Design review of the part built by this model. Coordinates are the model's own, in mm. A direction names the side the tool comes from. Give positions to 0.01 mm unless a question says otherwise; leave off trailing zeros. Loops run counter-clockwise (first coordinate to the right, second up) from the corner with the lowest first, then second, coordinate; pieces in that order, holes last. Notation, with made-up numbers: M 11,24 L 26,24 A28 cw 26,49 Z; hole C 37.25,6 d5. An arc over 180 degrees is marked long. Use a Markdown table: item, result. Add a question column.
(1) Add section C-C, the plane x = 7. Give the boundary of the cut face in (y, z).
(2) For faces 1 (the face through (0.507, -2.1, 0.5)), 2 (the face through (0.1, 3.954, 0.5)), list the 3-axis set-ups (+Z, -Z, +X, -X, +Y, -Y) from which the entire face can be reached by the end or side of a thin tool; tool diameter is ignored.
(3) Add section A-A, the plane x = 4.75. Give the boundary of the cut face in (y, z).
(4) Add section B-B, the plane y = -2.25. State how many separate pieces and enclosed holes the cut face has, then the cut area to 3 significant figures.
(5) For probe 1 along Y at (x, z) = (1.5, 0.6); probe 2 along Y at (x, z) = (3.5, 0.15); probe 3 along X at (y, z) = (-2.25, 0.5), list the stretches that pass through material, from the lowest coordinate up.
(6) Add section D-D, the plane z = 0.6. Give the boundary of the cut face in (x, y), then the cut area to 3 significant figures.
(7) Insertion check: pin 1 Ø0.5 at (y, z) = (-2.5, 0.5) entering from +X. The pin has a flat end and moves straight along its axis. Give the tip position at first contact, or say it passes through.
(8) Draft analysis for pull direction X (two halves, no side actions). For faces 3 (the face through (4.425, 1.184, 0.493)), 4 (the face through (-1, 0, 1)), 5 (the face through (8.036, -0.039, 0.699)), state which applies: pulls with the +X half, pulls with the -X half, needs draft (parallel to the pull), parting line crosses it, or undercut.
```python
from build123d import *

# Parameters (mm, degrees)
F1_DEPTH = 1
F2_R     = 0.99999


# Not quite as in the source:
# - a fillet or chamfer is up to 0.001 mm smaller than in the source, because OpenCascade refuses the exact size


with BuildPart() as f1:
    # F0 (on Top) → F1 (new body)
    with BuildSketch(Plane.XY):
        Polygon((-7.3084038651, 2.5000789639), (-8.3084038651, 2.9543336025), (-8.3084038651, -3.1456663975), (-7.3084038651, -2.6904001687), align=None)
        Polygon((-7.3084038651, 2.9543336025), (-8.3084038651, 2.9543336025), (-7.3084038651, 2.5000789639), align=None)
        Polygon((-7.3084038651, 3.9543336025), (-8.3084038651, 3.9543336025), (-8.3084038651, 2.9543336025), (-7.3084038651, 2.9543336025), (-5.1069954144, 2.9543336025), align=None)
        Polygon((-7.3084038651, -2.6904001687), (-8.3084038651, -3.1456663975), (-7.3084038651, -3.1456663975), align=None)
        Polygon((-7.3084038651, -3.1456663975), (-8.3084038651, -3.1456663975), (-8.3084038651, -4.1456663975), (-7.3017124087, -4.1456663975), (-5.1012464166, -3.1456663975), align=None)
        Polygon((-0.4934038651, -3.1456663975), (-5.1012464166, -3.1456663975), (-7.3017124087, -4.1456663975), (7.3215961349, -4.1456663975), (5.1201876842, -3.1456663975), (0.5065961349, -3.1456663975), align=None)
        Polygon((-7.3084038651, -2.6904001687), (-7.3084038651, -3.1456663975), (-5.1012464166, -3.1456663975), (-0.4934038651, -1.0516360566), (-0.4934038651, -0.5956663975), (-1.6015758867, -0.0922741165), align=None)
        Polygon((-0.0026520019, 0.6356619308), (-0.4934038651, 0.4122391807), (-0.4934038651, -0.5956663975), (0.0083764092, -0.8236024146), (0.5065961349, -0.597186861), (0.5065961349, 0.4043336025), align=None)
        Polygon((0.0083764092, -0.8236024146), (-0.4934038651, -0.5956663975), (-0.4934038651, -1.0516360566), align=None)
        Polygon((0.5065961349, -0.597186861), (0.0083764092, -0.8236024146), (0.5065961349, -1.0499210361), align=None)
        Polygon((1.6087379174, -0.0963194146), (0.5065961349, 0.4043336025), (0.5065961349, -0.597186861), align=None)
        Polygon((-0.0026520019, 0.6356619308), (-0.4934038651, 0.858588241), (-0.4934038651, 0.4122391807), align=None)
        Polygon((0.5065961349, 0.4043336025), (0.5065961349, 0.8675054096), (-0.0026520019, 0.6356619308), align=None)
        Polygon((0.5065961349, 2.9543336025), (-0.4934038651, 2.9543336025), (-0.4934038651, 0.858588241), (-0.0026520019, 0.6356619308), (0.5065961349, 0.8675054096), align=None)
        Polygon((-0.4934038651, -1.0516360566), (-0.4934038651, -3.1456663975), (0.5065961349, -3.1456663975), (0.5065961349, -1.0499210361), (0.0083764092, -0.8236024146), align=None)
        Polygon((7.3215961349, 2.9543336025), (5.0903496856, 2.9543336025), (0.5065961349, 0.8675054096), (0.5065961349, 0.4043336025), (1.6087379174, -0.0963194146), (7.3215961349, 2.4998844069), align=None)
        Polygon((8.3215961349, 3.9543336025), (7.2868666612, 3.9543336025), (5.0903496856, 2.9543336025), (7.3215961349, 2.9543336025), (8.3215961349, 2.9543336025), align=None)
        Polygon((7.3215961349, 2.4998844069), (8.3215961349, 2.9543336025), (7.3215961349, 2.9543336025), align=None)
        Polygon((8.3215961349, -3.1456663975), (8.3215961349, 2.9543336025), (7.3215961349, 2.4998844069), (7.3215961349, -2.691411759), align=None)
        Polygon((7.3215961349, -3.1456663975), (8.3215961349, -3.1456663975), (7.3215961349, -2.691411759), align=None)
        Polygon((8.3215961349, -4.1456663975), (8.3215961349, -3.1456663975), (7.3215961349, -3.1456663975), (5.1201876842, -3.1456663975), (7.3215961349, -4.1456663975), align=None)
        Polygon((-0.4934038651, 0.858588241), (-5.1069954144, 2.9543336025), (-7.3084038651, 2.9543336025), (-7.3084038651, 2.5000789639), (-1.6015758867, -0.0922741165), (-0.4934038651, 0.4122391807), align=None)
        Polygon((-0.4934038651, 0.4122391807), (-1.6015758867, -0.0922741165), (-0.4934038651, -0.5956663975), align=None)
        Polygon((5.1201876842, -3.1456663975), (7.3215961349, -3.1456663975), (7.3215961349, -2.691411759), (1.6087379174, -0.0963194146), (0.5065961349, -0.597186861), (0.5065961349, -1.0499210361), align=None)
        Polygon((7.2868666612, 3.9543336025), (-7.3084038651, 3.9543336025), (-5.1069954144, 2.9543336025), (-0.4934038651, 2.9543336025), (0.5065961349, 2.9543336025), (5.0903496856, 2.9543336025), align=None)
    extrude(amount=F1_DEPTH)

    # F2 (radius 1 in the source; OpenCascade refuses exactly that, so slightly less here)
    f2_edges = [f1.edges().sort_by_distance(p)[0] for p in [
        (8.321596, -0.095666, 1),
    ]]
    fillet(f2_edges, radius=F2_R)


solid = f1.part
```
Established:
| question | item | result |
|---|---|---|
| 1 | outline | M -4.15,0 L -2.55,0 L -2.55,1 L -4.15,1 Z; M 2.35,0 L 3.95,0 L 3.95,1 L 2.35,1 Z |
| 2 | face 1 | +Z, -Z |
| 2 | face 2 | +Z, -Z, +X, -X, +Y |
| 3 | outline | M -4.15,0 L -3.15,0 L -3.15,1 L -4.15,1 Z; M -2.98,0 L -1.52,0 L -1.52,1 L -2.98,1 Z; M 1.33,0 L 2.8,0 L 2.8,1 L 1.33,1 Z; M 2.95,0 L 3.95,0 L 3.95,1 L 2.95,1 Z |
| 4 | separate pieces | 5 |
| 4 | enclosed holes | 0 |
| 4 | area | 9.20 mm^2 |
| 5 | probe 1 | -4.15 to -3.15, -1.5 to 1.32, 2.95 to 3.95 |
| 5 | probe 2 | -4.15 to -3.15, -2.41 to -0.96, 0.76 to 2.23, 2.95 to 3.95 |
| 5 | probe 3 | -8.31 to -7.31, -6.34 to -3.13, -0.49 to 0.51, 3.15 to 6.35, 7.32 to 8.19 |
| 6 | outline | M -8.31,-4.15 L 8.12,-4.15 L 8.12,3.95 L -8.31,3.95 Z; hole M -7.31,-2.69 L -1.6,-0.09 L -7.31,2.5 Z; hole M -5.11,2.95 L -0.49,0.86 L -0.49,2.95 Z; hole M -5.1,-3.15 L -0.49,-3.15 L -0.49,-1.05 Z; hole M 0.51,-3.15 L 5.12,-3.15 L 0.51,-1.05 Z; hole M 0.51,0.87 L 5.09,2.95 L 0.51,2.95 Z; hole M 1.61,-0.1 L 7.32,-2.69 L 7.32,2.5 Z |
| 6 | area | 84.2 mm^2 |
| 7 | pin 1 | x = 8.29 |
| 8 | face 3 | undercut |
| 8 | face 4 | needs draft |
| 8 | face 5 | pulls with the +X half |
